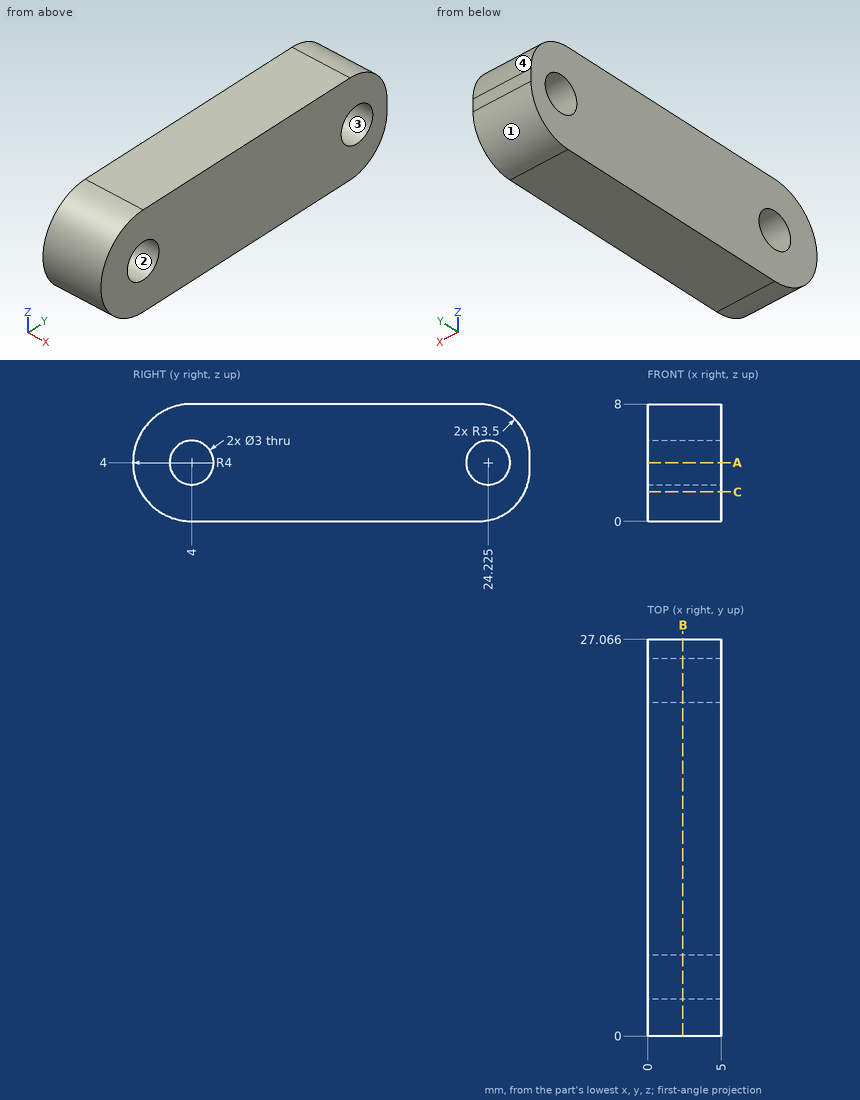
The drawing under review shows one solid part. Ordinate dimensions are in mm from its lowest x, y, z. Coordinates: 2 decimals unless noted, no trailing zeros. Order: outer loops, then holes, each group sorted by start corner. A loop starts at its lowest first (then second) coordinate and runs counter-clockwise, first axis right, second up. Notation, with made-up numbers: M 43.5,-17.75 L 70.5,-17.75 A13 ccw 70.5,4.25 Z; hole C 60.25,41.25 d7. An arc over 180 degrees is marked long. One line per question, with ' | ' between items.
(1) For probe 1 along Y at (x, z) = (3.6, 4) (1 decimal); probe 2 along Y at (x, z) = (2.95, 3.25) (1 decimal); probe 3 along Y at (x, z) = (2.15, 6.25), list the stretches that pass through material, from the lowest coordinate up. Write a range as from..to.
Geometry results:
probe 1: y = 0..2.5, 5.5..22.7, 25.7..27.1 | probe 2: y = 0.1..2.7, 5.3..22.9, 25.5..27.1 | probe 3: y = 0.69..26.6
(2) Add section A-A, the plane z = 4. Write out the cut boundary in (x, y) (1 decimal), then the cut area to 3 significant figures.
Geometry results:
outline: M 0,0 L 5,0 L 5,2.5 L 0,2.5 Z; M 0,5.5 L 5,5.5 L 5,22.7 L 0,22.7 Z; M 0,25.7 L 5,25.7 L 5,27.1 L 0,27.1 Z | area: 105 mm²
(3) Add section B-B, the plane x = 2.4. Write out the cut boundary in (y, z) (1 decimal).
Geometry results:
outline: M 4,0 L 23.6,0 A3.5 ccw 27.1,3.5 L 27.1,4.5 A3.5 ccw 23.6,8 L 4,8 A4 ccw Z; hole C 4,4 d3; hole C 24.2,4 d3
(4) The part is to be moulded in two halves that separate along Z. For the marked faces 1, 2, 3 and 4, say which applies: +Z half, -Z half, draft (parallel to the pull), parting line (faces both ways), or undercut.
Geometry results:
face 1: -Z half | face 2: undercut | face 3: undercut | face 4: +Z half
(5) Insertion check: pin 1 (1.5 mm diameter, centred on x = 3.5, z = 5.5, fed in from +Y); pin 2 (2 mm diameter, centred on x = 2, z = 2.5, fed in from -Y). Each pin has a flat end and moves straight along its axis. Give the tip position at first contact, or say it passes through.
Geometry results:
pin 1: stops at y = 27.06 | pin 2: stops at y = 0.03
(6) Add section C-C, the plane z = 2. Write out the cut boundary in (x, y), then the cut area to 3 significant figures.
Geometry results:
outline: M 0,0.54 L 5,0.54 L 5,26.73 L 0,26.73 Z | area: 131 mm²
